Work out the finished part from the listing and answer in its coordinate system (mm). Face numbers are marked on the shaded views. A direction names the side the tool comes from. Coordinates: 2 decimals unless noted, no trailing zeros. Write each loop counter-clockwise with the first axis right and the second up, starting at its lowest first coordinate (ties: lowest second). Pieces come first, ordered by that corner, then holes. Notation, with made-up numbers: (34, -39) - (56, -39) arc R12 cw to (56, -17) - close; hole circle Ø3 at (38, 87.25). An arc over 180 degrees is marked (long way). Use one line per item in the form item = value. Start each with the question number.
Item 1: Given pin 1 (2.5 mm diameter, centred on x = 17, y = 7, fed in from +Z); pin 2 (6 mm diameter, centred on x = 15, y = 10.5, fed in from -Z); pin 3 (3.5 mm diameter, centred on x = 0, z = -10, fed in from -Y); pin 4 (1 mm diameter, centred on y = 9.5, z = -7.5, fed in from -X), each flat-ended and moving along its own axis, determine where each tip first touches the part or whether it passes through.
Item 2: Consider probe 1 along Z at (x, y) = (14, 9); probe 2 along Y at (x, z) = (2.75, -11); probe 3 along Y at (x, z) = (11, -8.25). Determine where each line is inside the solid, lowest interval first.
Item 3: A cutting plane is placed at C-C (z = -9). Write down the section's boundary in (x, y), then the cut area to 3 significant figures.
Item 4: For the marked faces 4 and 5, determine the directions among +Z, -Z, +X, -X, +Y, -Y from which every point of the face is accessible in a straight line to the end or side of a thin tool.
Item 5: Determine the mould class of the marked faces 1, 2 and 3 for opening direction X: released by +X, released by -X, zero draft, split by the parting line, or undercut.
Item 6: A cutting plane is placed at A-A (y = 4). Write down the section's boundary in (x, z) (3 decimals).
Item 7: A cutting plane is placed at B-B (x = 0). Write down the section's boundary in (y, z), then the cut area to 3 significant figures.
Item 8: A cutting plane is placed at D-D (y = 8.7). Write down the section's boundary in (x, z) (3 decimals).
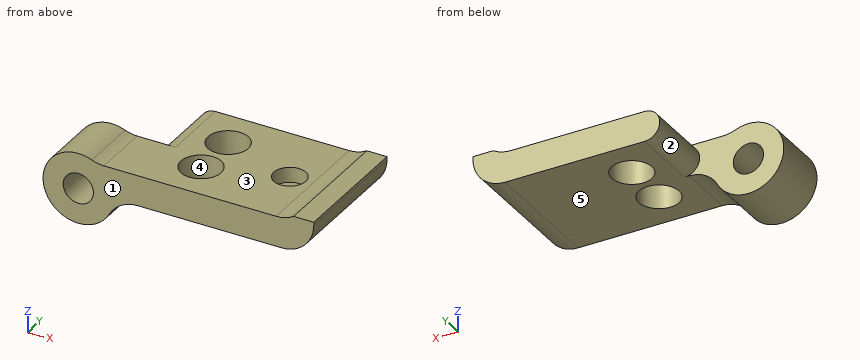
from build123d import *

# Parameters (mm, degrees)
SKETCH1_R           = 3.5
BOSS_EXTRUDE1_DEPTH = 12.7
CUT_EXTRUDE1_DEPTH  = 6.93
SKETCH3_R           = 1.5
CUT_EXTRUDE2_DEPTH  = 6.77
SKETCH4_R           = 2
CUT_EXTRUDE3_DEPTH  = 10
SKETCH5_W           = 2
SKETCH5_H           = 0.5
BOSS_EXTRUDE2_DEPTH = 12.7
FILLET1_R           = 3.175
SKETCH6_R           = 1.585
CUT_EXTRUDE4_DEPTH  = 1.5


with BuildPart() as part:
    # Sketch1 → Boss-Extrude1 (new body)
    with BuildSketch(Plane(origin=(0, 0, 0), x_dir=(1, 0, 0), z_dir=(0, 1, 0))):
        Circle(SKETCH1_R)
        with BuildLine():
            ThreePointArc((1.802775638, 3), (3.046285831, 1.723410176), (3.5, 0))
            Line((3.5, 0), (23.330212793, 0))
            Line((23.330212793, 0), (23.330212793, 3))
            Line((23.330212793, 3), (1.802775638, 3))
        make_face()
    extrude(amount=BOSS_EXTRUDE1_DEPTH)

    # Sketch2 → Cut-Extrude1 (cut)
    with BuildSketch(Plane(origin=(0, 12.7, 0), x_dir=(1, 0, 0), z_dir=(0, 1, 0))):
        with BuildLine():
            ThreePointArc((6.330212793, 3), (-6.149926342, 1.5), (6.330212793, 0))
            Line((6.330212793, 0), (3.5, 0))
            ThreePointArc((3.5, 0), (-3.046285831, -1.723410176), (1.802775638, 3))
            Line((1.802775638, 3), (6.330212793, 3))
        make_face()
        with BuildLine():
            Line((3.5, 0), (6.330212793, 0))
            ThreePointArc((6.330212793, 0), (4.830212793, 1.5), (6.330212793, 3))
            Line((6.330212793, 3), (1.802775638, 3))
            ThreePointArc((1.802775638, 3), (-3.046285831, -1.723410176), (3.5, 0))
        make_face()
    extrude(amount=-CUT_EXTRUDE1_DEPTH, mode=Mode.SUBTRACT)

    # Sketch3 → Cut-Extrude2 (cut, through all)
    with BuildSketch(Plane(origin=(0, 5.77, 0), x_dir=(1, 0, 0), z_dir=(0, 1, 0))):
        with Locations(Location((0, 0, 0), (0, 0, 270))):  # turned: the seam where the file's is
            Circle(SKETCH3_R)
    extrude(amount=-CUT_EXTRUDE2_DEPTH, mode=Mode.SUBTRACT)


with BuildPart() as body_2:
    # Mirror1: mirrored copy
    add(part.part.mirror(Plane.XY.offset(-5)))

    # Sketch4 → Cut-Extrude3 (cut)
    with BuildSketch(Plane.XY.offset(-7)):
        with Locations((9.871541535, 8.7)):
            Circle(SKETCH4_R)
        with Locations((9.871541535, 4)):
            Circle(SKETCH4_R)
    extrude(amount=-CUT_EXTRUDE3_DEPTH, mode=Mode.SUBTRACT)

    # Sketch5 → Boss-Extrude2 (add)
    with BuildSketch(Plane(origin=(0, 12.7, 0), x_dir=(1, 0, 0), z_dir=(0, 1, 0))):
        with BuildLine():
            Line((21.330212793, 6.5), (21.330212793, 7))
            Line((21.330212793, 7), (19.59096008, 7))
            ThreePointArc((19.59096008, 7), (20.495808134, 6.872518864), (21.330212793, 6.5))
        make_face()
        with Locations((22.330212793, 6.75)):
            Rectangle(SKETCH5_W, SKETCH5_H)
    extrude(amount=-BOSS_EXTRUDE2_DEPTH)

    # Fillet1
    fillet1_edges = [body_2.edges().sort_by_distance(p)[0] for p in [
        (1.802775638, 2.885, -7),
        (3.5, 2.885, -10),
        (23.330212793, 6.35, -10),
    ]]
    fillet(fillet1_edges, radius=FILLET1_R)

    # Sketch6 → Cut-Extrude4 (cut)
    with BuildSketch(Plane.XY.offset(-7)):
        with Locations((17.330212793, 6.35)):
            Circle(SKETCH6_R)
    extrude(amount=-CUT_EXTRUDE4_DEPTH, mode=Mode.SUBTRACT)


solid = body_2.part
Answer:
q1.pin_1 = -7
q1.pin_2 = -10
q1.pin_3 = 0
q1.pin_4 = 4.92
q2.probe_1 = -10 to -7
q2.probe_2 = 0 to 5.77
q2.probe_3 = 0 to 2.35, 5.65 to 7.05, 10.35 to 12.7
q3.outline = (-3.35, 0) - (-1.12, 0) - (-1.12, 5.77) - (-3.35, 5.77) - close; (1.12, 0) - (22.47, 0) - (22.47, 12.7) - (4.92, 12.7) - (4.92, 5.77) - (1.12, 5.77) - close; hole circle Ø4 at (9.87, 4); hole circle Ø4 at (9.87, 8.7)
q3.area = 233 mm²
q4.face_4 = +Z, -Z
q4.face_5 = -Z, +X, +Y, -Y
q5.face_1 = zero draft
q5.face_2 = released by -X
q5.face_3 = undercut
q6.outline = (1.329, -6.762) arc R3.5 ccw (long way) to (3.079, -11.665) arc R3.175 cw to (5.872, -10) - (7.872, -10) - (7.872, -7) - (2.535, -7) arc R3.175 cw to start; (11.872, -10) - (20.155, -10) arc R3.175 ccw to (23.33, -6.825) - (23.33, -6.5) - (21.33, -6.5) arc R3.275 cw to (19.591, -7) - (11.872, -7) - close; hole circle Ø3 at (0, -10)
q7.outline = (0, -13.5) - (5.77, -13.5) - (5.77, -11.5) - (0, -11.5) - close; (0, -8.5) - (5.77, -8.5) - (5.77, -6.5) - (0, -6.5) - close
q7.area = 23.1 mm²
q8.outline = (6.33, -10) - (7.872, -10) - (7.872, -7) - (6.33, -7) arc R1.5 ccw to start; (11.872, -10) - (20.155, -10) arc R3.175 ccw to (23.33, -6.825) - (23.33, -6.5) - (21.33, -6.5) arc R3.275 cw to (19.591, -7) - (11.872, -7) - close
